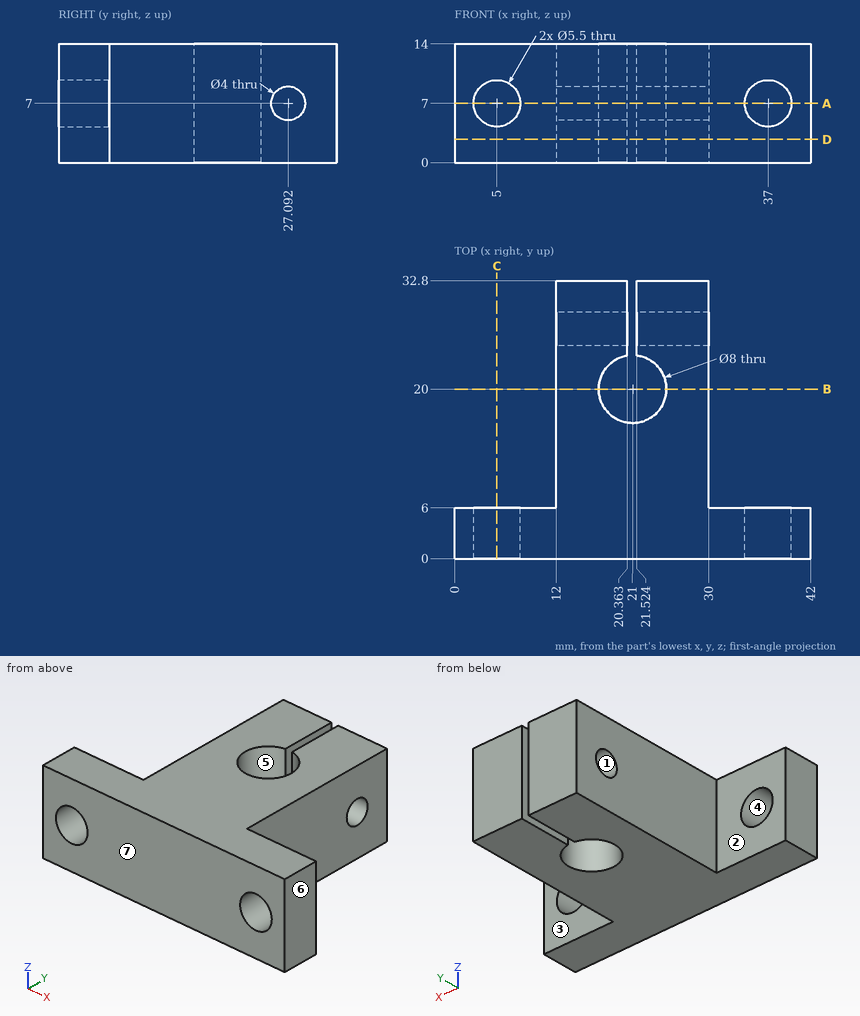
Check sheet for the drawn part. Datum: minimum x, y, z corner. Units: mm. A direction names the side the tool comes from. Round coordinates to 2 decimals unless told otherwise and drop trailing zeros. Loops run counter-clockwise (first coordinate to the right, second up) from the corner with the lowest first, then second, coordinate; pieces in that order, holes last. Notation, with made-up numbers: M 44.25,-29.5 L 102.25,-29.5 A26 cw 102.25,7.5 Z; hole C 9,36 d10. An arc over 180 degrees is marked long. One line per question, with ' | ' between items. Start each with the question number.
Item 1: Release check for a two-part mould opening along X. For the marked faces 4, 5, 6 and 7 record: released by +X, released by -X, zero draft, split by the parting line, or undercut.
Item 2: Section check A-A (z = 7). State how many separate pieces and enclosed holes the cut face has.
Item 3: Set-up check for the marked faces 1, 2 and 3: record each of +Z, -Z, +X, -X, +Y, -Y from which the full face is reachable in a straight line by a thin tool's end or side.
Item 4: Section check C-C (x = 5). Record the boundary of the cut face in (y, z).
Item 5: Gauge pin test, flat ends, axial feed: pin 1 Ø4 at (y, z) = (22.5, 9.5) entering from +X; pin 2 Ø8 at (x, y) = (14.5, 10) entering from -Z; pin 3 Ø4 at (y, z) = (15.5, 6.5) entering from -X; pin 4 Ø3.5 at (x, z) = (36, 8) entering from +Y. Record the tip position at first contact, or that the pin passes through.
Item 6: Section check D-D (z = 2.75). Record the boundary of the cut face in (x, y) (1 decimal).
Item 7: Scan lines: probe 1 along X at (y, z) = (1.35, 7); probe 2 along X at (y, z) = (31.5, 6.5) (1 decimal); probe 3 along Y at (x, z) = (17.5, 7) (1 decimal). Record each from-to range of solid material in increasing order.
Item 8: Section check B-B (y = 20). Record the boundary of the cut face in (x, z).
Worked out:
1) face 4: undercut | face 5: undercut | face 6: released by +X | face 7: zero draft
2) separate pieces: 5 | enclosed holes: 0
3) face 1: +X, -X | face 2: +Z, -Z, -X, +Y | face 3: +Z, -Z, +X, +Y
4) outline: M 0,0 L 6,0 L 6,4.25 L 0,4.25 Z; M 0,9.75 L 6,9.75 L 6,14 L 0,14 Z
5) pin 1: x = 30 | pin 2: z = 0 | pin 3: x = 12 | pin 4: y = 6
6) outline: M 0,0 L 42,0 L 42,6 L 30,6 L 30,32.8 L 21.5,32.8 L 21.5,24 A4 cw long 20.4,23.9 L 20.4,32.8 L 12,32.8 L 12,6 L 0,6 Z
7) probe 1: 0 to 2.25, 7.75 to 34.25, 39.75 to 42 | probe 2: 12 to 20.4, 21.5 to 30 | probe 3: 0 to 18.1, 21.9 to 25.1, 29.1 to 32.8
8) outline: M 12,0 L 17,0 L 17,14 L 12,14 Z; M 25,0 L 30,0 L 30,14 L 25,14 Z
